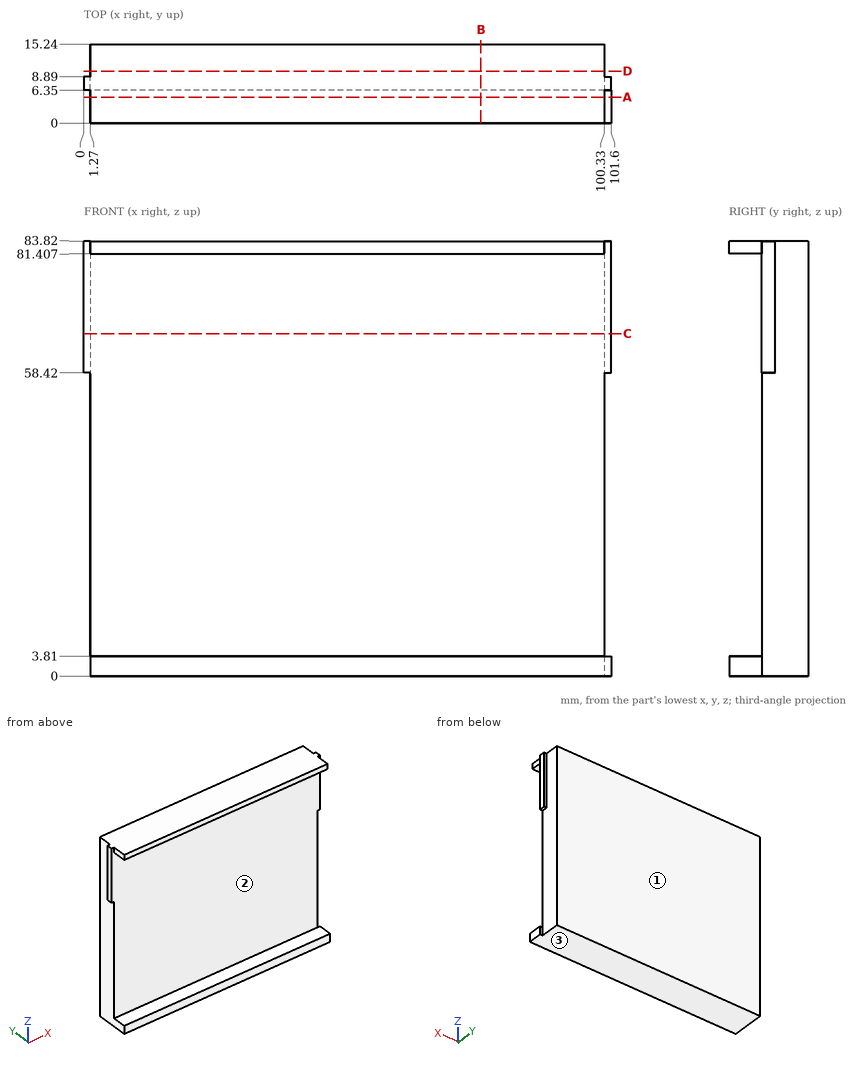
For this review, use the dimensioned drawing (mm, ordinates from the lowest corner) and the shaded views. Give positions to 0.01 mm unless a question says otherwise; leave off trailing zeros. Loops run counter-clockwise (first coordinate to the right, second up) from the corner with the lowest first, then second, coordinate; pieces in that order, holes last. Notation, with made-up numbers: (1.25, 64) -> (51.25, 64) arc R34 ccw to (51.25, 102) -> close; hole circle Ø10 at (75.5, 64). An arc over 180 degrees is marked (long way). One line per question, with ' | ' between items. Start each with the question number.
(1) For line 1 (Z direction, x = 88.5, y = 3.5); line 2 (Y direction, x = 7.5, z = 15); line 3 (X direction, y = 9.5, z = 70), list the stretches that pass through material, from the lowest coordinate up.
(2) Insertion check: P1, Ø1, axis at x = 0.5, z = 71, coming from the +Y side; P2, Ø1.9, axis at y = 2.5, z = 83, coming from the +X side; P3, Ø1, axis at x = 90, z = 67, coming from the -Y side; P4, Ø7, axis at x = 43.5, y = 2.5, coming from the -Z side. Each pin has a flat end and moves straight along its axis. Give the tip position at first contact, or say it passes through.
(3) We need section B-B (x = 76.5). State the section outline as (y, z) points, and give its area (3 significant figures).
(4) We need section C-C (z = 66). State the section outline as (x, y) points.
(5) Draft analysis for pull direction Z (two halves, no side actions). For the marked faces 1, 2 and 3, state which applies: +Z half, -Z half, draft (parallel to the pull), parting line (faces both ways), or undercut.
(6) We need section A-A (y = 5). State the section outline as (x, z) points.
(7) We need section D-D (y = 10). State the section outline as (x, z) points.
The answers:
1) line 1: z = 0 to 3.81, 81.41 to 83.82 | line 2: y = 6.35 to 15.24 | line 3: x = 1.27 to 100.33
2) P1: stops at y = 8.89 | P2: stops at x = 100.33 | P3: stops at y = 6.35 | P4: stops at z = 0
3) outline: (0, 0) -> (15.24, 0) -> (15.24, 83.82) -> (0, 83.82) -> (0, 81.41) -> (6.35, 81.41) -> (6.35, 3.81) -> (0, 3.81) -> close | area: 785 mm^2
4) outline: (0, 6.35) -> (101.6, 6.35) -> (101.6, 8.89) -> (100.33, 8.89) -> (100.33, 15.24) -> (1.27, 15.24) -> (1.27, 8.89) -> (0, 8.89) -> close
5) face 1: draft | face 2: undercut | face 3: -Z half
6) outline: (1.27, 0) -> (101.6, 0) -> (101.6, 3.81) -> (1.27, 3.81) -> close; (1.27, 81.41) -> (100.33, 81.41) -> (100.33, 83.82) -> (1.27, 83.82) -> close
7) outline: (1.27, 0) -> (100.33, 0) -> (100.33, 83.82) -> (1.27, 83.82) -> close
